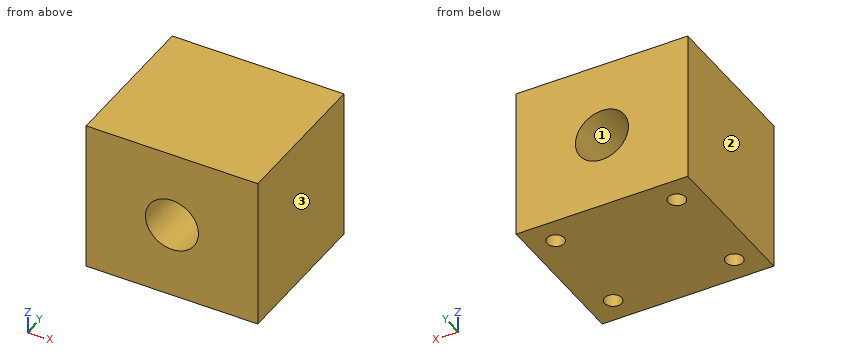
```python
from build123d import *

# Parameters (mm, degrees)
SKETCH_1_W               = 34
SKETCH_1_H               = 30
EXTRUDE_1_DEPTH          = 30
CUT_EXTRUDE_1_DEPTH      = 55.369108876
CUT_EXTRUDE_1_DEPTH_BACK = 55.369108876
SKETCH_2_R               = 5.25
SKETCH_3_R               = 1.7
CUT_EXTRUDE_2_DEPTH      = 4


with BuildPart() as part:
    # 草图1 → 凸台-拉伸1 (new body)
    with BuildSketch(Plane.XY):
        with Locations((17, 15)):
            Rectangle(SKETCH_1_W, SKETCH_1_H)
    extrude(amount=EXTRUDE_1_DEPTH)

    # 草图2 → 切除-拉伸1 (cut, two sides: drawn at the far end of the back side and taken through both)
    with BuildSketch(Plane(origin=(0, 30, 0), x_dir=(1, 0, 0), z_dir=(0, 1, 0)).offset(-CUT_EXTRUDE_1_DEPTH_BACK)):
        with Locations(Location((17, -15, 0), (0, 0, 270))):
            Circle(SKETCH_2_R)
    extrude(amount=CUT_EXTRUDE_1_DEPTH + CUT_EXTRUDE_1_DEPTH_BACK, mode=Mode.SUBTRACT)

    # 草图3 → 切除-拉伸2 (cut)
    with BuildSketch(Plane(origin=(0, 0, 0), x_dir=(-1, 0, 0), z_dir=(0, 0, -1))):
        with Locations((-29, 25)):
            Circle(SKETCH_3_R)
        with Locations(Location((-29, 5, 0), (0, 0, 180))):
            Circle(SKETCH_3_R)
        with Locations((-5, 5)):
            Circle(SKETCH_3_R)
        with Locations(Location((-5, 25, 0), (0, 0, 180))):
            Circle(SKETCH_3_R)
    extrude(amount=-CUT_EXTRUDE_2_DEPTH, mode=Mode.SUBTRACT)


solid = part.part
```
Geometry: final body of the model. Coordinates: model frame, mm. Face numbers are marked on the shaded views. Round coordinates to 2 decimals unless told otherwise and drop trailing zeros. Loops run counter-clockwise (first coordinate to the right, second up) from the corner with the lowest first, then second, coordinate; pieces in that order, holes last.
Item 1: Section D-D, the plane z = 2. Output: boundary loops of the cut face in (x, y).
Checked values:
outline: (0, 0) - (34, 0) - (34, 30) - (0, 30) - close; hole circle Ø3.4 at (5, 5); hole circle Ø3.4 at (5, 25); hole circle Ø3.4 at (29, 5); hole circle Ø3.4 at (29, 25)
Item 2: Mould query, pull axis X, two halves, no side actions, for the marked faces 1, 2 and 3. Classes: released by +X, released by -X, zero draft, split by the parting line, or undercut.
Checked values:
face 1: undercut
face 2: released by -X
face 3: released by +X
Item 3: Section B-B, the plane y = 25. Output: boundary loops of the cut face in (x, z), plus the area to 3 significant figures.
Checked values:
outline: (0, 0) - (3.3, 0) - (3.3, 4) - (6.7, 4) - (6.7, 0) - (27.3, 0) - (27.3, 4) - (30.7, 4) - (30.7, 0) - (34, 0) - (34, 30) - (0, 30) - close; hole circle Ø10.5 at (17, 15)
area: 906 mm2
Item 4: Section A-A, the plane z = 15. Output: boundary loops of the cut face in (x, y).
Checked values:
outline: (0, 0) - (11.75, 0) - (11.75, 30) - (0, 30) - close; (22.25, 0) - (34, 0) - (34, 30) - (22.25, 30) - close
Item 5: Line query: L1, parallel to Y at x = 29, z = 1.25; L2, parallel to Z at x = 16.5, y = 26; L3, parallel to X at y = 11.5, z = 16.5. Output: solid intervals per line, ascending.
Checked values:
L1: y = 0 to 3.3, 6.7 to 23.3, 26.7 to 30
L2: z = 0 to 9.77, 20.23 to 30
L3: x = 0 to 11.97, 22.03 to 34
Item 6: Contact query for a flat-ended pin moving along its axis: P1, Ø1, axis at x = 30, y = 5.5, coming from the -Z side. Output: stop coordinate, or through.
Checked values:
P1: stops at z = 4
Item 7: Section C-C, the plane x = 29. Output: boundary loops of the cut face in (y, z).
Checked values:
outline: (0, 0) - (3.3, 0) - (3.3, 4) - (6.7, 4) - (6.7, 0) - (23.3, 0) - (23.3, 4) - (26.7, 4) - (26.7, 0) - (30, 0) - (30, 30) - (0, 30) - close
